Drawing for the job (mm, zero at the part's lowest x, y, z). A direction names the side the tool comes from. Coordinates: 2 decimals unless noted, no trailing zeros. Order: outer loops, then holes, each group sorted by start corner. A loop starts at its lowest first (then second) coordinate and runs counter-clockwise, first axis right, second up.
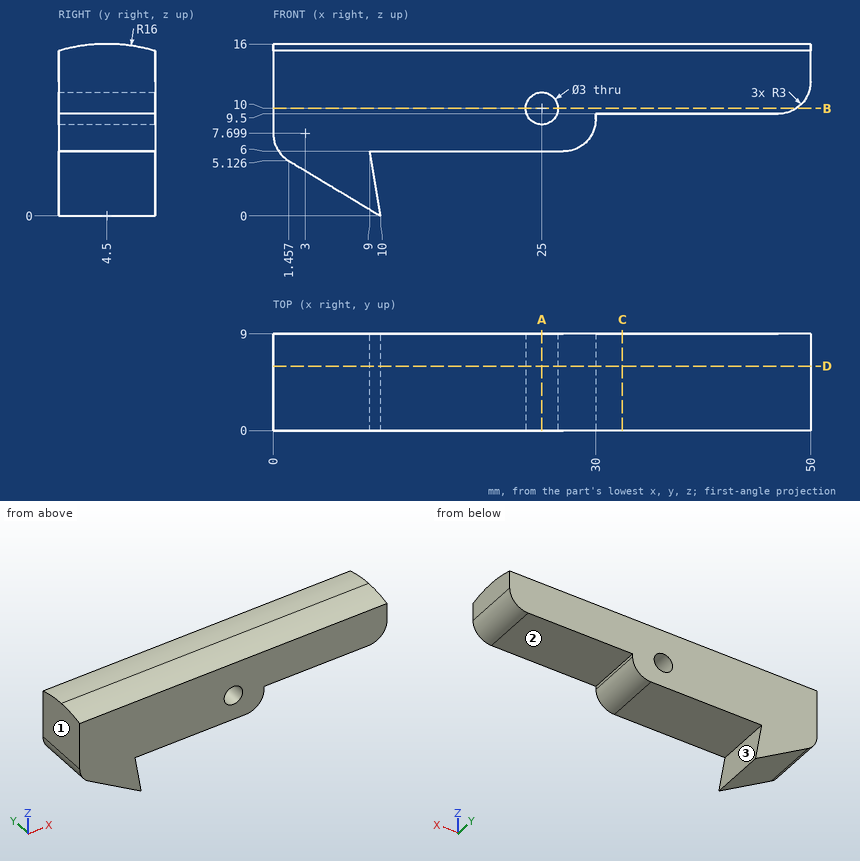
(1) Probe line 1 (X direction, y = 3, z = 10) (1 decimal); line 2 (Z direction, x = 18.5, y = 4.25); line 3 (Z direction, x = 32, y = 4.5). List the from-to ranges inside material, lowest first.
(2) Drop flat-ended pins along their axis: pin 1 (4 mm diameter, centred on x = 26, y = 4.5, fed in from -Z); pin 2 (5 mm diameter, centred on x = 19.5, y = 8, fed in from +Z); pin 3 (5 mm diameter, centred on y = 6.5, z = 4.5, fed in from +X) (1 decimal). Give the stop position or say it passes through.
(3) Slice it at A-A, the plane x = 25. Give the cut face in (y, z) (1 decimal).
(4) Slice it at C-C, the plane x = 32.5. Give the cut face in (y, z) (1 decimal).
(5) Tool access for the marked faces 1, 2 and 3: list every direction of +Z, -Z, +X, -X, +Y, -Y with a clear straight run to the whole face (end or side of a thin tool).
(6) Slice it at D-D, the plane y = 6. Give the cut face in (x, z), then the cut area to 3 significant figures.
(7) Slice it at B-B, the plane z = 10. Give the cut face in (x, y).
Here are the results:
1. line 1: x = 0 to 23.5, 26.5 to 48.7
1. line 2: z = 6 to 16
1. line 3: z = 9.5 to 16
2. pin 1: stops at z = 6
2. pin 2: stops at z = 15.97
2. pin 3: stops at x = 29.2
3. outline: (0, 6) - (9, 6) - (9, 8.5) - (0, 8.5) - close; (0, 11.5) - (9, 11.5) - (9, 15.4) arc R16 ccw to (0, 15.4) - close
4. outline: (0, 9.5) - (9, 9.5) - (9, 15.4) arc R16 ccw to (0, 15.4) - close
5. face 1: +Z, -Z, -X, +Y, -Y
5. face 2: -Z, +X, +Y, -Y
5. face 3: +X, +Y, -Y
6. outline: (0, 7.7) arc R3 ccw to (1.46, 5.13) - (10, 0) - (9, 6) - (27, 6) arc R3 ccw to (30, 9) - (30, 9.5) - (47, 9.5) arc R3 ccw to (50, 12.5) - (50, 15.93) - (0, 15.93) - close; hole circle Ø3 at (25, 10)
6. area: 442 mm2
7. outline: (0, 0) - (23.5, 0) - (23.5, 9) - (0, 9) - close; (26.5, 0) - (48.66, 0) - (48.66, 9) - (26.5, 9) - close
